CAD build for the part. Positions are in the model's coordinates, mm. Face numbers are marked on the shaded views. Give positions to 0.01 mm unless a question says otherwise; leave off trailing zeros. Order: outer loops, then holes, each group sorted by start corner. A loop starts at its lowest first (then second) coordinate and runs counter-clockwise, first axis right, second up. Notation, with made-up numbers: (37, 26.5) -> (47, 26.5) arc R13 ccw to (47, 41.5) -> close; hole circle Ø4 at (65.5, 30). An arc over 180 degrees is marked (long way). Answer as CSV lines item,"result".
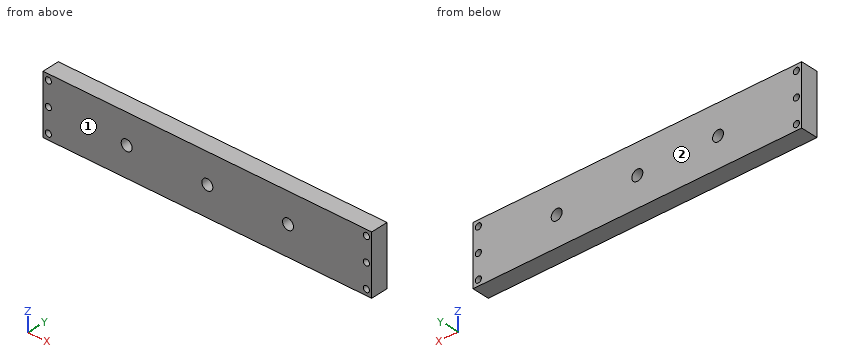
```python
from build123d import *

# Parameters (mm, degrees)
SKETCH1_W           = 203.2
SKETCH1_H           = 36.79952
BOSS_EXTRUDE1_DEPTH = 10.668
SKETCH3_R           = 1.905
CUT_EXTRUDE1_DEPTH  = 11.668
SKETCH4_R           = 3.3782
CUT_EXTRUDE2_DEPTH  = 11.668


with BuildPart() as part:
    # Sketch1 → Boss-Extrude1 (new body)
    with BuildSketch(Plane(origin=(0, 0, 0), x_dir=(1, 0, 0), z_dir=(0, 1, 0))):
        Rectangle(SKETCH1_W, SKETCH1_H)
    extrude(amount=BOSS_EXTRUDE1_DEPTH)

    # Sketch3 → Cut-Extrude1 (cut, through all)
    with BuildSketch(Plane.XZ):
        with Locations((-98.298, 14.732)):
            Circle(SKETCH3_R)
        with Locations((-98.298, 0)):
            Circle(SKETCH3_R)
        with Locations((-98.298, -14.732)):
            Circle(SKETCH3_R)
    cut_extrude1 = extrude(amount=-CUT_EXTRUDE1_DEPTH, mode=Mode.SUBTRACT)

    # Mirror1: Cut-Extrude1 across plane
    add(cut_extrude1.mirror(Plane(origin=(0, 0, 0), x_dir=(0, 0, 1), z_dir=(1, 0, 0))), mode=Mode.SUBTRACT)

    # Sketch4 → Cut-Extrude2 (cut, through all)
    with BuildSketch(Plane(origin=(0, 10.668, 0), x_dir=(1, 0, 0), z_dir=(0, 1, 0))):
        with Locations((-49.8856, 0)):
            Circle(SKETCH4_R)
        Circle(SKETCH4_R)
        with Locations((49.8856, 0)):
            Circle(SKETCH4_R)
    extrude(amount=-CUT_EXTRUDE2_DEPTH, mode=Mode.SUBTRACT)


solid = part.part
```
1) Band-saw the part on A-A, the plane z = 0. Write the cut outline in (x, y), then the cut area to 3 significant figures.
Data:
outline,"(-101.6, 0) -> (-100.2, 0) -> (-100.2, 10.67) -> (-101.6, 10.67) -> close; (-96.39, 0) -> (-53.26, 0) -> (-53.26, 10.67) -> (-96.39, 10.67) -> close; (-46.51, 0) -> (-3.38, 0) -> (-3.38, 10.67) -> (-46.51, 10.67) -> close; (3.38, 0) -> (46.51, 0) -> (46.51, 10.67) -> (3.38, 10.67) -> close; (53.26, 0) -> (96.39, 0) -> (96.39, 10.67) -> (53.26, 10.67) -> close; (100.2, 0) -> (101.6, 0) -> (101.6, 10.67) -> (100.2, 10.67) -> close"
area,"1,870 mm2"
2) Band-saw the part on B-B, the plane x = 0. Write the cut outline in (y, z), then the cut area to 4 significant figures.
Data:
outline,"(0, -18.4) -> (10.67, -18.4) -> (10.67, -3.38) -> (0, -3.38) -> close; (0, 3.38) -> (10.67, 3.38) -> (10.67, 18.4) -> (0, 18.4) -> close"
area,"320.5 mm2"
3) Wall check: line 1 along X through (y, z) = (1.75, -15); line 2 along X through (y, z) = (9.5, -0.5); line 3 along X through (y, z) = (4.25, 13.5) (3 decimals). Give the ranges that are in metal, low to high. Write a range as [from, to].
Data:
line 1,"x = [-101.6, -100.18], [-96.41, 96.41], [100.18, 101.6]"
line 2,"x = [-101.6, -100.14], [-96.46, -53.23], [-46.54, -3.34], [3.34, 46.54], [53.23, 96.46], [100.14, 101.6]"
line 3,"x = [-101.6, -99.751], [-96.845, 96.845], [99.751, 101.6]"
4) Band-saw the part on C-C, the plane y = 3.75. Give the number of separate pieces and of enclosed holes in the cut face, then the cut area to 3 significant figures.
Data:
separate pieces,"1"
enclosed holes,"9"
area,"7,300 mm2"
5) Pull direction Y, two halves, no side cores. Call the marked faces 1 and 2: pulls with the +Y half, pulls with the -Y half, needs draft (parallel to the pull), parting line crosses it, or undercut.
Data:
face 1,"pulls with the -Y half"
face 2,"pulls with the +Y half"
6) Pin check, flat tip, straight feed: P1, Ø3.5, axis at x = -98.298, z = 14.732, coming from the +Y side. Stop position of the tip, or through.
Data:
P1,"passes through"
